```python
from build123d import *

# Parameters (mm, degrees)
PAD005_DEPTH    = 10
SKETCH010_R     = 3
SKETCH010_R_2   = 3.175
POCKET005_DEPTH = 10.001
SKETCH011_R     = 1.7
POCKET006_DEPTH = 10.001
POCKET004_DEPTH = 4.5


with BuildPart() as part:
    # Sketch012 → Pad005 (new body)
    with BuildSketch(Plane.XY):
        with BuildLine():
            Line((-10.5, 0), (10.5, 0))
            ThreePointArc((13.5, -3), (12.62132, -0.87868), (10.5, 0))
            Line((13.5, -3), (13.5, -22))
            ThreePointArc((10.5, -25), (12.62132, -24.12132), (13.5, -22))
            Line((10.5, -25), (-10.5, -25))
            ThreePointArc((-13.5, -22), (-12.62132, -24.12132), (-10.5, -25))
            Line((-13.5, -22), (-13.5, -3))
            ThreePointArc((-10.5, 0), (-12.62132, -0.87868), (-13.5, -3))
        make_face()
    extrude(amount=PAD005_DEPTH)

    # Sketch010 → Pocket005 (cut, through all)
    with BuildSketch(Plane.XY):
        with Locations((0, -7)):
            Circle(SKETCH010_R)
        with Locations((0, -15.5)):
            Circle(SKETCH010_R_2)
    extrude(amount=POCKET005_DEPTH, mode=Mode.SUBTRACT)

    # Sketch011 → Pocket006 (cut, through all)
    with BuildSketch(Plane.XY):
        with Locations((-10, -4.2)):
            Circle(SKETCH011_R)
        with Locations((10, -4.2)):
            Circle(SKETCH011_R)
    extrude(amount=POCKET006_DEPTH, mode=Mode.SUBTRACT)

    # Sketch013 → Pocket004 (cut)
    with BuildSketch(Plane.XY):
        with BuildLine():
            Line((-6.75, 5), (-6.75, -5))
            ThreePointArc((-9.75, -8), (-7.62868, -7.12132), (-6.75, -5))
            Line((-9.75, -8), (-20, -8))
            Line((-20, -8), (-20, 10))
            Line((-20, 10), (20, 10))
            Line((20, 10), (20, -8))
            Line((20, -8), (9.75, -8))
            ThreePointArc((6.75, -5), (7.62868, -7.12132), (9.75, -8))
            Line((6.75, -5), (6.75, 5))
            Line((6.75, 5), (-6.75, 5))
        make_face()
    extrude(amount=POCKET004_DEPTH, mode=Mode.SUBTRACT)


with BuildPart() as part_1:
    # Body004 placement: moved
    add(part.part.moved(Location((0, -1, -25))))


solid = part_1.part
```
Build history of the part. All positions in model axes, mm. A direction names the side the tool comes from. Give positions to 0.01 mm unless a question says otherwise; leave off trailing zeros. Order: outer loops, then holes, each group sorted by start corner. A loop starts at its lowest first (then second) coordinate and runs counter-clockwise, first axis right, second up. Notation, with made-up numbers: M 35,74 L 79,74 A21 cw 79,98 Z; hole C 62.25,43.5 d2. An arc over 180 degrees is marked long. Return JSON: item names as keys, results as strings.
Q1. 3-axis set-ups, long thin cutter, end or side, ignore diameter. For faces 1 (the face through (3.03, -15.55, -20.07)), 2 (the face through (6.75, -4, -23)), 3 (the face through (-6.75, -3, -23)): which of +Z, -Z, +X, -X, +Y, -Y reach the whole face in a straight line?
Answer list:
{"face 1": "+Z, -Z", "face 2": "-Z, +X, +Y", "face 3": "-Z, -X, +Y"}
Q2. Flat gauge pins, fed straight in: pin 1 (5.5 mm diameter, centred on x = -11.5, y = -6, fed in from -Z); pin 2 (1.3 mm diameter, centred on y = -4, z = -24, fed in from -X); pin 3 (2 mm diameter, centred on y = -2.5, z = -23, fed in from +X). Where does each tip first touch, or does it go through?
Answer list:
{"pin 1": "stops at z = -20.5", "pin 2": "stops at x = -6.75", "pin 3": "stops at x = 6.75"}
Q3. Wall check: probe 1 along Y at (x, z) = (0, -22.5) (3 decimals); probe 2 along Y at (x, z) = (-0.5, -17); probe 3 along X at (y, z) = (-8, -19.5). Give the ranges that are in metal, low to high. Write a range as from..to.
Answer list:
{"probe 1": "y = -26..-19.675, -13.325..-11, -5..-1", "probe 2": "y = -26..-19.64, -13.36..-10.96, -5.04..-1", "probe 3": "x = -13.5..-3, 3..13.5"}
Q4. Band-saw the part on C-C (x = -2). Give the cut face in (y, z), then the cut area to 3 significant figures.
Answer list:
{"outline": "M -26,-25 L -18.97,-25 L -18.97,-15 L -26,-15 Z; M -14.03,-25 L -10.24,-25 L -10.24,-15 L -14.03,-15 Z; M -5.76,-25 L -1,-25 L -1,-15 L -5.76,-15 Z", "area": "156 mm^2"}
Q5. Band-saw the part on A-A (z = -22.25). Give the cut face in (x, y) (3 decimals), then the cut area to 3 significant figures.
Answer list:
{"outline": "M -13.5,-23 A3 ccw -10.5,-26 L 10.5,-26 A3 ccw 13.5,-23 L 13.5,-9 L 9.75,-9 A3 cw 6.75,-6 L 6.75,-1 L -6.75,-1 L -6.75,-6 A3 cw -9.75,-9 L -13.5,-9 Z; hole C 0,-16.5 d6.35; hole C 0,-8 d6", "area": "507 mm^2"}
Q6. Band-saw the part on D-D (x = -9). Give the cut face in (y, z), then the cut area to 3 significant figures.
Answer list:
{"outline": "M -26,-25 L -8.9,-25 L -8.9,-20.5 L -6.57,-20.5 L -6.57,-15 L -26,-15 Z; M -3.83,-20.5 L -1,-20.5 L -1,-15 L -3.83,-15 Z", "area": "199 mm^2"}
Q7. Two-plate mould, pull along Y, no slides. Class faces 4 (the face through (-13.5, -14, -20)), 5 (the face through (-12, -9, -23)), 6 (the face through (-8.43, -5.85, -17.79)): pulls with the +Y half, pulls with the -Y half, needs draft (parallel to the pull), parting line crosses it, or undercut.
Answer list:
{"face 4": "needs draft", "face 5": "pulls with the +Y half", "face 6": "undercut"}
Q8. Band-saw the part on B-B (y = -16.5). Give the cut face in (x, z) (3 decimals).
Answer list:
{"outline": "M -13.5,-25 L -3.175,-25 L -3.175,-15 L -13.5,-15 Z; M 3.175,-25 L 13.5,-25 L 13.5,-15 L 3.175,-15 Z"}
